Source: CAD feature listing. Evaluate the final solid. Frame: model axes, mm. A direction names the side the tool comes from. Coordinates: 2 decimals unless noted, no trailing zeros. Loops run counter-clockwise (first coordinate to the right, second up) from the corner with the lowest first, then second, coordinate; pieces in that order, holes last. Notation, with made-up numbers: M -1.75,55.25 L 9.25,55.25 A37 ccw 9.25,94.25 Z; hole C 82,15.25 d6. An arc over 180 degrees is marked long. Write each question's results on one line, items separated by ' | '. Start each with the question number.
Autodesk Inventor part; units mm, degrees
ref_plane "YZ Plane" through (0, 0, 0) normal (1, 0, 0) x (0, 1, 0)
ref_plane "XZ Plane" through (0, 0, 0) normal (0, 1, 0) x (-1, 0, 0)
ref_plane "XY Plane" through (0, 0, 0) normal (0, 0, 1) x (1, 0, 0)
sketch "Esboço1" plane through (0, 0, 0) normal (0, 0, 1) x (1, 0, 0)
  line L0 (-70.9188, 104.3152) -> (40.0812, 104.3152)
  line L1 (-70.9188, 5.5999) -> (-70.9188, 104.3152)
  line L2 (-24.6341, -40.6848) -> (86.1475, -40.6848)
  line L3 (86.1475, -40.6848) -> (86.1475, -0.6848)
  line L4 (86.1475, -0.6848) -> (40.0812, -0.6848)
  line L5 (40.0812, -0.6848) -> (40.0812, 104.3152)
  line L6 (-24.6341, -40.6848) -> (-70.9188, 5.5999)
  line L7 (-24.6341, -40.6848) -> (40.8222, -40.6848) construction
  point P0 (0, 0)
  dimension "d0" = 111
  dimension "d5" = 40
  dimension "d6" = 105
  dimension "d7" = 135
  dimension "d8" = 98.7154
  dimension "d11" = 157.0662
extrude "Extrusão1" add sketch "Esboço1" along normal blind 12.7
chamfer "Chanfro1" distance 20 angle 45 1 edges at (-70.9188, 104.3152, 6.35)
sketch "Esboço2" plane through (0, 0, 12.7) normal (0, 0, 1) x (1, 0, 0)
  circle A0 centre (-45.7988, 78.3152) radius 2.75 construction
  circle A1 centre (-63.7988, 78.3152) radius 2.75 construction
  circle A2 centre (-45.7988, 32.3152) radius 2.75 construction
  circle A3 centre (-63.7988, 32.3152) radius 2.75 construction
  point P0 (0, 0)
hole "Furo1" at (-45.7988, 78.3152, 12.7) at (-63.7988, 78.3152, 12.7) at (-45.7988, 32.3152, 12.7) at (-63.7988, 32.3152, 12.7) direction (0, 0, -1) diameter 4.134 end through all
sketch "Esboço3" plane through (0, 0, 0) normal (0, 0, -1) x (-1, 0, 0)
  line L0 (30.2988, 72.8152) -> (61.2988, 72.8152)
  line L1 (63.2988, 70.8152) -> (63.2988, 39.8152)
  line L2 (61.2988, 37.8152) -> (30.2988, 37.8152)
  line L3 (28.2988, 39.8152) -> (28.2988, 70.8152)
  line L4 (28.2988, 72.8152) -> (63.2988, 37.8152) construction
  line L5 (63.2988, 72.8152) -> (28.2988, 37.8152) construction
  arc A0 (30.2988, 72.8152) -> (28.2988, 70.8152) centre (30.2988, 70.8152) ccw
  arc A1 (28.2988, 39.8152) -> (30.2988, 37.8152) centre (30.2988, 39.8152) ccw
  arc A2 (61.2988, 37.8152) -> (63.2988, 39.8152) centre (61.2988, 39.8152) ccw
  arc A3 (63.2988, 70.8152) -> (61.2988, 72.8152) centre (61.2988, 70.8152) ccw
  point P0 (0, 0)
  dimension "d22" = 35
  dimension "d23" = 35
  dimension "d24" = 2
extrude "Extrusão2" cut sketch "Esboço3" against normal through all
sketch "Esboço4" plane through (0, 0, 0) normal (0, 0, -1) x (-1, 0, 0)
  circle A0 centre (-12.5812, 19.3152) radius 4
  circle A1 centre (-12.5812, -20.6848) radius 4
  line L0 (-40.0812, 104.3152) -> (-40.0812, -0.6848)
  line L1 (-86.1475, -40.6848) -> (24.6341, -40.6848)
  point P0 (0, 0)
  point P1 (-12.5812, 19.3152)
  point P2 (-12.5812, -20.6848)
  dimension "d27" = 8
  dimension "d28" = 8
  dimension "d36" = 27.5
  dimension "d37" = 60
  dimension "d38" = 20
  dimension "d39" = 27.5
hole "Furo2" at (12.5812, 19.3152, 0) at (12.5812, -20.6848, 0) direction (0, 0, 1) diameter 8.5 end through all
sketch "Esboço5" plane through (0, 0, 0) normal (0, 0, -1) x (-1, 0, 0)
  line L0 (-86.1475, -16.2848) -> (-33.1475, -16.2848) construction
  line L1 (-86.1475, -25.0848) -> (-33.1475, -25.0848) construction
  line L2 (-59.6475, -16.2848) -> (-59.6475, -25.0848) construction
  line L3 (-33.1475, -16.2848) -> (-33.1475, -25.0848) construction
  line L4 (-86.1475, -0.6848) -> (-86.1475, -41.0283) construction
  line L5 (-46.3975, -16.2848) -> (-46.3975, -25.0848) construction
  line L6 (-72.8975, -16.2848) -> (-72.8975, -25.0848) construction
  line L7 (-33.1475, -20.6848) -> (-86.1475, -20.6848) construction
  line L8 (-86.1475, -0.6848) -> (-86.1475, -40.6848)
  circle A0 centre (-46.3975, -20.6848) radius 2.5 construction
  circle A1 centre (-72.8975, -20.6848) radius 2.5 construction
  point P0 (0, 0)
  dimension "d40" = 26.5
  dimension "d41" = 13.25
  dimension "d42" = 13.25
  dimension "d43" = 53
  dimension "d44" = 5
  dimension "d45" = 5
hole "Furo3" at (72.8975, -20.6848, 0) at (46.3975, -20.6848, 0) direction (0, 0, 1) diameter 5.5 end through all
equation "\"d41\" = 0.5 * d40"
equation "\"d42\" = d41"
properties part number "SUPORTE_MANCAL_TRASEIRO"
Item 1: Cut plane C-C (y = 11). Output: boundary loops of the cut face in (x, z), then the cut area to 3 significant figures.
Item 2: Mould query, pull axis X, two halves, no side actions, for faces 4 (the flat face through (-70.919, 44, 6)), 5 (the flat face through (63, -0.685, 6)), 6 (the cylindrical face through (-45.89, 80.38, 6.26)). Classes: +X half, -X half, draft (parallel to the pull), parting line (faces both ways), or undercut.
Item 3: Cut plane A-A (x = -33). Output: boundary loops of the cut face in (y, z).
Item 4: Line query: probe 1 along Y at (x, z) = (12, 4.5); probe 2 along Y at (x, z) = (-63.5, 12.25); probe 3 along X at (y, z) = (31, 2.75). Output: solid intervals per line, ascending.
Item 5: Access query for faces 1 (the flat face through (30, -40.685, 6)), 2 (the flat face through (-46, 72.815, 6)), 3 (the flat face through (40.081, 51, 6)). Directions: +Z, -Z, +X, -X, +Y, -Y. A direction counts if a zero-diameter tool reaches every point of the face in a straight line with its end or side. Return the directions, or none.
Item 6: Cut plane B-B (z = 10). Count the separate pieces of the cut face and the enclosed holes in it, then the cut area to 3 significant figures.
Item 7: Cut plane D-D (x = 68). Output: boundary loops of the cut face in (y, z).
Item 8: First-contact query: pin 1 Ø1.5 at (x, y) = (-19.5, 89.5) entering from -Z; pin 2 Ø4 at (x, z) = (-39.5, 3.5) entering from -Y; pin 3 Ø6.5 at (x, z) = (57, 8.5) entering from +Y. Flat tips, straight axial feed; report the tip coordinate or a pass-through.
Response values:
1) outline: M -70.92,0 L 40.08,0 L 40.08,12.7 L -70.92,12.7 Z | area: 1,410 mm2
2) face 4: -X half | face 5: draft | face 6: undercut
3) outline: M -32.32,0 L 37.82,0 L 37.82,12.7 L -32.32,12.7 Z; M 72.82,0 L 104.32,0 L 104.32,12.7 L 72.82,12.7 Z
4) probe 1: y = -40.68 to -24.89, -16.47 to 15.11, 23.53 to 104.32 | probe 2: y = -1.82 to 30.27, 34.36 to 76.27, 80.36 to 91.73 | probe 3: x = -70.92 to -65.39, -62.2 to -47.39, -44.2 to 40.08
5) face 1: +Z, -Z, +X, -X, -Y | face 2: +Z, -Z | face 3: +Z, -Z, +X, +Y
6) separate pieces: 1 | enclosed holes: 9 | area: 15,200 mm2
7) outline: M -40.68,0 L -0.68,0 L -0.68,12.7 L -40.68,12.7 Z
8) pin 1: stops at z = 0 | pin 2: stops at y = -27.82 | pin 3: stops at y = -0.68
